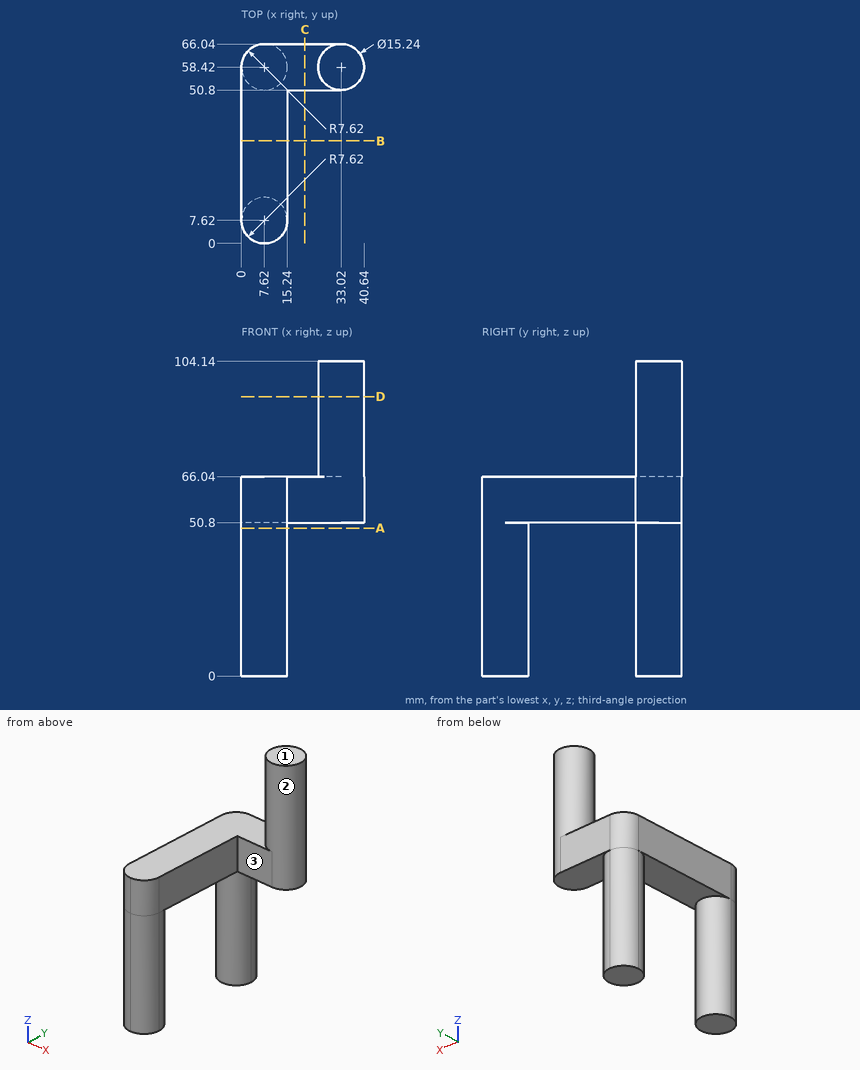
Could you check a few things on this drawing? It's one solid part, dimensions in mm from its lowest x, y, z. A direction names the side the tool comes from. Coordinates: 2 decimals unless noted, no trailing zeros. Order: outer loops, then holes, each group sorted by start corner. A loop starts at its lowest first (then second) coordinate and runs counter-clockwise, first axis right, second up. Notation, with made-up numbers: (58.25, -24) -> (76.25, -24) arc R13 cw to (76.25, -11) -> close; hole circle Ø7 at (14.5, 2). An arc over 180 degrees is marked (long way). One line per item, written item: value. Start each with the question number.
1) Imagine slicing it at B-B on y = 34. List the corners of the cut face in (x, z) for me, plus the area to 3 significant figures.
2) If I drill on L1, parallel to Z at x = 20, y = 59; L2, parallel to X at y = 48, z = 57.5; L3, parallel to Z at x = 8, y = 58, over which ranges is the centre line in solid material (lowest first)? Write a range as [from, to].
3) Imagine slicing it at C-C on x = 21. List the corners of the cut face in (y, z) for me.
4) Which directions (+Z, -Z, +X, -X, +Y, -Y) give clear straight access to the entire face, cutting with the end or side of a thin tool? Please do the marked faces 1, 2 and 3.
5) Imagine slicing it at A-A on z = 49. List the corners of the cut face in (x, y) for me.
6) Imagine slicing it at D-D on z = 92.5. List the corners of the cut face in (x, y) for me, plus the area to 3 significant figures.
7) I'm going to push flat-ended pins straight in: pin 1 (5 mm diameter, centred on x = 4, z = 35.5, fed in from +Y); pin 2 (3 mm diameter, centred on x = 13.5, z = 18, fed in from -Y); pin 3 (1.5 mm diameter, centred on x = 6.5, z = 42.5, fed in from -Y). Where does each tip first touch, or does it pass through?
Answer list:
1. outline: (0, 50.8) -> (15.24, 50.8) -> (15.24, 66.04) -> (0, 66.04) -> close
1. area: 232 mm2
2. L1: z = [50.8, 66.04]
2. L2: x = [0, 15.24]
2. L3: z = [0, 66.04]
3. outline: (50.8, 50.8) -> (66.04, 50.8) -> (66.04, 66.04) -> (50.8, 66.04) -> close
4. face 1: +Z, +X, -X, +Y, -Y
4. face 2: +Z
4. face 3: +Z, -Z, +X, -Y
5. outline: circle Ø15.24 at (7.62, 7.62); circle Ø15.24 at (7.62, 58.42)
6. outline: circle Ø15.24 at (33.02, 58.42)
6. area: 182 mm2
7. pin 1: stops at y = 65.96
7. pin 2: stops at y = 1.38
7. pin 3: stops at y = 0.01
